from build123d import *

# Parameters (mm, degrees)
SKETCH1_W                        = 150
SKETCH1_H                        = 190
BOSS_EXTRUDE1_DEPTH              = 6
SKETCH2_W                        = 30
SKETCH2_H                        = 18.75
CUT_EXTRUDE1_DEPTH               = 6
CHAMFER1_SIZE                    = 5
SKETCH3_W                        = 20
SKETCH3_H                        = 40
CUT_EXTRUDE2_DEPTH               = 6
SKETCH5_R                        = 1.125
CUT_EXTRUDE4_DEPTH               = 3.75
SKETCH9_R                        = 5
POLE_SUPPORTS_DEPTH              = 17.5
FILLET1_R                        = 5
SKETCH10_R                       = 3.5
POLE_SUPPORT_HOLE_LEFT_DEPTH     = 17.5
SKETCH11_R                       = 3.5
POLE_SUPPORT_HOLE_RIGHT_DEPTH    = 17.5
SKETCH12_R                       = 2
POLE_SUPPORT_SCREW_DEPTH         = 6
SKETCH13_W                       = 42
SKETCH13_H                       = 30.4
PULLEY_MOUNT_DEPTH               = 1.8
SKETCH15_R                       = 1.5
PULLEY_MOUNT_SCREWS_DEPTH        = 4.7
SKETCH16_W                       = 4
SKETCH16_H                       = 49
MOTOR_MOUNTS_DEPTH               = 49
SKETCH17_R                       = 7
SKETCH17_R_2                     = 1.5
MOTOR_MOUNTING_HOLES_LEFT_DEPTH  = 4
SKETCH18_W                       = 29
SKETCH18_H                       = 41
MOTOR_CUTOUT_LEFT_DEPTH          = 6.5
FILLET2_R                        = 2.5
MOTOR_START                      = -4
SKETCH20_R                       = 7
SKETCH20_R_2                     = 1.5
MOTOR_MOUNTING_HOLES_RIGHT_DEPTH = 4
SKETCH21_W                       = 29
SKETCH21_H                       = 41
MOTOR_CUTOUT_RIGHT_DEPTH         = 6
FILLET3_R                        = 2.5
SKETCH23_R                       = 1.5
ARDUINO_MOUNTING_HOLES_DEPTH     = 6
SKETCH24_R                       = 4
CUT_EXTRUDE20_DEPTH              = 2
CHAMFER2_SIZE                    = 5
FILLET4_R                        = 3.5


with BuildPart() as part:
    # Sketch1 → Boss-Extrude1 (new body)
    with BuildSketch(Plane(origin=(0, 0, 0), x_dir=(1, 0, 0), z_dir=(0, 1, 0))):
        Rectangle(SKETCH1_W, SKETCH1_H)
    extrude(amount=BOSS_EXTRUDE1_DEPTH)

    # Sketch2 → Cut-Extrude1 (cut)
    with BuildSketch(Plane(origin=(0, 6, 0), x_dir=(1, 0, 0), z_dir=(0, 1, 0))):
        with Locations((-60, 85.625)):
            Rectangle(SKETCH2_W, SKETCH2_H)
        with Locations((60, 85.625)):
            Rectangle(SKETCH2_W, SKETCH2_H)
    extrude(amount=-CUT_EXTRUDE1_DEPTH, mode=Mode.SUBTRACT)

    # Chamfer1
    chamfer1_edges = [part.edges().sort_by_distance(p)[0] for p in [
        (-75, 3, -76.25),
        (-45, 3, -95),
        (75, 3, -76.25),
        (45, 3, -95),
    ]]
    chamfer(chamfer1_edges, length=CHAMFER1_SIZE)

    # Sketch3 → Cut-Extrude2 (cut)
    with BuildSketch(Plane(origin=(0, 6, 0), x_dir=(1, 0, 0), z_dir=(0, 1, 0))):
        with Locations((-65, -75)):
            Rectangle(SKETCH3_W, SKETCH3_H)
        with Locations((65, -75)):
            Rectangle(SKETCH3_W, SKETCH3_H)
    extrude(amount=-CUT_EXTRUDE2_DEPTH, mode=Mode.SUBTRACT)

    # Sketch5 → Cut-Extrude4 (cut)
    with BuildSketch(Plane(origin=(0, 6, 0), x_dir=(1, 0, 0), z_dir=(0, 1, 0))):
        with Locations(Location((0, -74, 0), (0, 0, 270))):
            Circle(SKETCH5_R)
        with Locations(Location((0, -35.7, 0), (0, 0, 270))):
            Circle(SKETCH5_R)
    extrude(amount=-CUT_EXTRUDE4_DEPTH, mode=Mode.SUBTRACT)

    # Sketch9 → Pole supports (add)
    with BuildSketch(Plane(origin=(0, 6, 0), x_dir=(1, 0, 0), z_dir=(0, 1, 0))):
        with Locations(Location((-45, 58.865040338, 0), (0, 0, 270))):
            Circle(SKETCH9_R)
        with Locations(Location((45, 58.865040338, 0), (0, 0, 270))):
            Circle(SKETCH9_R)
    extrude(amount=POLE_SUPPORTS_DEPTH)

    # Fillet1
    fillet1_edges = [part.edges().sort_by_distance(p)[0] for p in [
        (-45, 6, -63.865040338),
        (45, 6, -63.865040338),
    ]]
    fillet(fillet1_edges, radius=FILLET1_R)

    # Sketch10 → Pole support hole - left (cut)
    with BuildSketch(Plane(origin=(0, 23.5, 0), x_dir=(1, 0, 0), z_dir=(0, 1, 0))):
        with Locations(Location((-45, 58.865040338, 0), (0, 0, 270))):
            Circle(SKETCH10_R)
    extrude(amount=-POLE_SUPPORT_HOLE_LEFT_DEPTH, mode=Mode.SUBTRACT)

    # Sketch11 → Pole support hole - right (cut)
    with BuildSketch(Plane(origin=(0, 23.5, 0), x_dir=(1, 0, 0), z_dir=(0, 1, 0))):
        with Locations(Location((45, 58.865040338, 0), (0, 0, 270))):
            Circle(SKETCH11_R)
    extrude(amount=-POLE_SUPPORT_HOLE_RIGHT_DEPTH, mode=Mode.SUBTRACT)

    # Sketch12 → Pole support screw (cut)
    with BuildSketch(Plane(origin=(0, 6, 0), x_dir=(1, 0, 0), z_dir=(0, 1, 0))):
        with Locations(Location((-45, 58.865040338, 0), (0, 0, 270))):
            Circle(SKETCH12_R)
        with Locations(Location((45, 58.865040338, 0), (0, 0, 270))):
            Circle(SKETCH12_R)
    extrude(amount=-POLE_SUPPORT_SCREW_DEPTH, mode=Mode.SUBTRACT)

    # Sketch13 → Pulley mount (cut)
    with BuildSketch(Plane(origin=(0, 6, 0), x_dir=(1, 0, 0), z_dir=(0, 1, 0))):
        with Locations((29.5, 22.18)):
            Rectangle(SKETCH13_W, SKETCH13_H)
    extrude(amount=-PULLEY_MOUNT_DEPTH, mode=Mode.SUBTRACT)

    # Sketch15 → Pulley mount screws (cut)
    with BuildSketch(Plane(origin=(0, 4.2, 0), x_dir=(1, 0, 0), z_dir=(0, 1, 0))):
        with Locations(Location((13.9, 34.68, 0), (0, 0, 270))):
            Circle(SKETCH15_R)
        with Locations(Location((46.5, 34.68, 0), (0, 0, 270))):
            Circle(SKETCH15_R)
        with Locations(Location((46.5, 9.68, 0), (0, 0, 270))):
            Circle(SKETCH15_R)
        with Locations(Location((13.9, 9.68, 0), (0, 0, 270))):
            Circle(SKETCH15_R)
    extrude(amount=-PULLEY_MOUNT_SCREWS_DEPTH, mode=Mode.SUBTRACT)

    # Sketch16 → Motor mounts (add)
    with BuildSketch(Plane(origin=(0, 6, 0), x_dir=(1, 0, 0), z_dir=(0, 1, 0))):
        with Locations((-73, -30.5)):
            Rectangle(SKETCH16_W, SKETCH16_H)
        with Locations((73, -30.5)):
            Rectangle(SKETCH16_W, SKETCH16_H)
    extrude(amount=MOTOR_MOUNTS_DEPTH)

    # Sketch17 → Motor mounting holes - left (cut)
    with BuildSketch(Plane(origin=(-71, 0, 0), x_dir=(0, 0, -1), z_dir=(1, 0, 0))):
        with Locations((-30.5, 18.5)):
            Circle(SKETCH17_R)
        with Locations((-39.5, 9.5)):
            Circle(SKETCH17_R_2)
        with Locations((-21.5, 9.5)):
            Circle(SKETCH17_R_2)
        with Locations((-39.5, 42.5)):
            Circle(SKETCH17_R_2)
        with Locations((-21.5, 42.5)):
            Circle(SKETCH17_R_2)
    extrude(amount=-MOTOR_MOUNTING_HOLES_LEFT_DEPTH, mode=Mode.SUBTRACT)

    # Sketch18 → Motor cutout - left (cut)
    with BuildSketch(Plane(origin=(0, 6, 0), x_dir=(1, 0, 0), z_dir=(0, 1, 0))):
        with Locations((-56.5, -30.5)):
            Rectangle(SKETCH18_W, SKETCH18_H)
    extrude(amount=-MOTOR_CUTOUT_LEFT_DEPTH, mode=Mode.SUBTRACT)

    # Fillet2
    fillet2_edges = [part.edges().sort_by_distance(p)[0] for p in [
        (-71, 6, 53),
        (-71, 6, 8),
    ]]
    fillet(fillet2_edges, radius=FILLET2_R)

    # Sketch20 → Motor mounting holes - right (cut)
    with BuildSketch(Plane.ZY.offset(-71).offset(MOTOR_START)):
        with Locations(Location((30.5, 18.5, 0), (0, 0, 180))):
            Circle(SKETCH20_R)
        with Locations(Location((21.5, 9.5, 0), (0, 0, 180))):
            Circle(SKETCH20_R_2)
        with Locations(Location((39.5, 9.5, 0), (0, 0, 180))):
            Circle(SKETCH20_R_2)
        with Locations(Location((21.5, 42.5, 0), (0, 0, 180))):
            Circle(SKETCH20_R_2)
        with Locations(Location((39.5, 42.5, 0), (0, 0, 180))):
            Circle(SKETCH20_R_2)
    extrude(amount=MOTOR_MOUNTING_HOLES_RIGHT_DEPTH, mode=Mode.SUBTRACT)

    # Sketch21 → Motor cutout - right (cut)
    with BuildSketch(Plane(origin=(0, 6, 0), x_dir=(1, 0, 0), z_dir=(0, 1, 0))):
        with Locations((56.5, -30.5)):
            Rectangle(SKETCH21_W, SKETCH21_H)
    extrude(amount=-MOTOR_CUTOUT_RIGHT_DEPTH, mode=Mode.SUBTRACT)

    # Fillet3
    fillet3_edges = [part.edges().sort_by_distance(p)[0] for p in [
        (71, 6, 8),
        (71, 6, 53),
    ]]
    fillet(fillet3_edges, radius=FILLET3_R)

    # Sketch23 → Arduino mounting holes (cut)
    with BuildSketch(Plane(origin=(0, 6, 0), x_dir=(1, 0, 0), z_dir=(0, 1, 0))):
        with Locations(Location((-27.5, -6.754956847, 0), (0, 0, 270))):
            Circle(SKETCH23_R)
        with Locations(Location((27.5, -6.754956847, 0), (0, 0, 270))):
            Circle(SKETCH23_R)
        with Locations(Location((-27.5, -80, 0), (0, 0, 270))):
            Circle(SKETCH23_R)
        with Locations(Location((27.5, -80, 0), (0, 0, 270))):
            Circle(SKETCH23_R)
    extrude(amount=-ARDUINO_MOUNTING_HOLES_DEPTH, mode=Mode.SUBTRACT)

    # Sketch24 → Cut-Extrude20 (cut)
    with BuildSketch(Plane.XZ):
        with Locations(Location((45, -58.865040338, 0), (0, 0, 270))):
            Circle(SKETCH24_R)
        with Locations(Location((-45, -58.865040338, 0), (0, 0, 270))):
            Circle(SKETCH24_R)
    extrude(amount=-CUT_EXTRUDE20_DEPTH, mode=Mode.SUBTRACT)

    # Chamfer2
    chamfer2_edges = [part.edges().sort_by_distance(p)[0] for p in [
        (-55, 3, 95),
        (55, 3, 95),
    ]]
    chamfer(chamfer2_edges, length=CHAMFER2_SIZE)

    # Fillet4
    fillet4_edges = [part.edges().sort_by_distance(p)[0] for p in [
        (-42, 3, 10),
        (-42, 3, 51),
        (42, 3, 51),
        (42, 3, 10),
    ]]
    fillet(fillet4_edges, radius=FILLET4_R)


solid = part.part
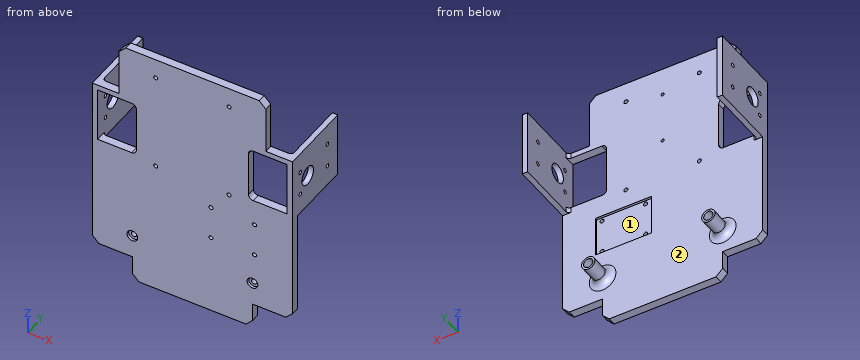
Could you check a few things on this model? Use its own coordinates, in mm. Face numbers are marked on the shaded views. Give positions to 0.01 mm unless a question says otherwise; leave off trailing zeros. Order: outer loops, then holes, each group sorted by start corner. A loop starts at its lowest first (then second) coordinate and runs counter-clockwise, first axis right, second up. Notation, with made-up numbers: (23.5, -40) - (34.5, -40) arc R23 ccw to (34.5, -26) - close; hole circle Ø7 at (70, -20.5). An arc over 180 degrees is marked (long way). One line per question, with ' | ' between items. Start each with the question number.
Item 1: I want a section at B-B on x = 61.5. Write out the boundary of the cut face in (y, z), then the cut area to 4 significant figures.
Item 2: I'm going to push flat-ended pins straight in: pin 1 Ø6 at (x, y) = (-66.5, 20.5) entering from +Z; pin 2 Ø5 at (x, z) = (43, -58) entering from +Y; pin 3 Ø3.5 at (x, z) = (-45, -59.5) entering from +Y; pin 4 Ø5 at (x, y) = (-71.5, 32) entering from -Z. Where does each tip first touch, or does it pass through?
Item 3: I want a section at A-A on y = 37. Write out the boundary of the cut face in (x, z).
Item 4: Thinking about a two-plate mould opening in Z: for the marked faces 1 and 2, which applies, pulls with the +Z half, pulls with the -Z half, needs draft (parallel to the pull), parting line crosses it, or undercut?
Item 5: I want a section at D-D on x = 18. Write out the boundary of the cut face in (y, z), then the cut area to 3 significant figures.
Item 6: I want a section at C-C on z = 30.5. Write out the boundary of the cut face in (x, y).
Item 7: I need wall thicknesses on probe 1 along Y at (x, z) = (73.55, 39.5); probe 2 along X at (y, z) = (38, 34.5); probe 3 along Z at (x, y) = (27, 2). Which ranges of each line are inside material? Lowest first, please. Write a range as [from, to].
Verdict:
1) outline: (0, -76.25) - (6, -76.25) - (6, 10) - (0, 10) - close; (0, 51) - (6, 51) - (6, 55) - (0, 55) - close | area: 541.5 mm^2
2) pin 1: through | pin 2: y = 23.5 | pin 3: y = 6 | pin 4: z = 6
3) outline: (-75, 6) - (-71, 6) - (-71, 55) - (-75, 55) - close; (71, 6) - (75, 6) - (75, 55) - (71, 55) - close
4) face 1: undercut | face 2: needs draft
5) outline: (0, -95) - (6, -95) - (6, -37.38) - (4.2, -37.38) - (4.2, -6.98) - (6, -6.98) - (6, 95) - (0, 95) - close | area: 1,090 mm^2
6) outline: (-75, 0) - (-71, 0) - (-71, 11.5) - (-75, 11.5) - close; (-75, 25.5) - (-71, 25.5) - (-71, 55) - (-75, 55) - close; (-42, 0) - (42, 0) - (42, 6) - (-42, 6) - close; (71, 0) - (75, 0) - (75, 11.5) - (71, 11.5) - close; (71, 25.5) - (75, 25.5) - (75, 55) - (71, 55) - close
7) probe 1: [0, 8], [11, 41], [44, 55] | probe 2: [-75, -71], [71, 75] | probe 3: [-95, 5.34], [8.17, 78.59], [81.41, 95]
